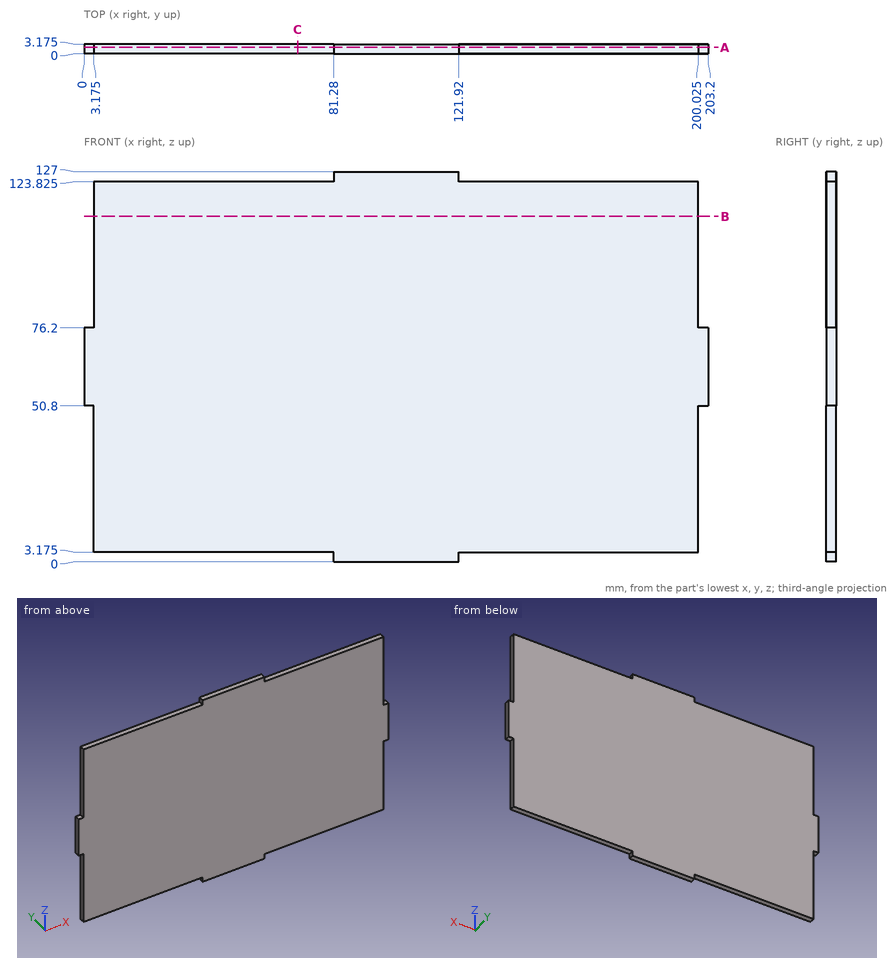
Part print with two shaded views. Sizes in mm from the minimum x, y, z corner. Coordinates: 2 decimals unless noted, no trailing zeros. Write each loop counter-clockwise with the first axis right and the second up, starting at its lowest first coordinate (ties: lowest second). Pieces come first, ordered by that corner, then holes.
(1) Pin check, flat tips, straight feed: pin 1 Ø8 at (x, z) = (45, 27.5) entering from -Y; pin 2 Ø1 at (x, y) = (31.5, 1.5) entering from -Z (3 decimals); pin 3 Ø1 at (x, y) = (2, 1) entering from +Z; pin 4 Ø1 at (y, z) = (1, 1.5) entering from +X. Stop position of each tip, or through.
(2) Cut at A-A on y = 2.1. List the corners of the cut face in (x, z) (3 decimals).
(3) Cut at C-C on x = 69.5. List the corners of the cut face in (y, z) (3 decimals), and give its area (3 significant figures).
(4) Cut at B-B on z = 112.5. List the corners of the cut face in (x, y) (3 decimals).
(5) Drill centre lines: line 1 (Z direction, x = 190, y = 1.75) (3 decimals); line 2 (X direction, y = 2.3, z = 46) (3 decimals). Where is each one in solid material? Low to high.
Working result:
1. pin 1: stops at y = 0
1. pin 2: stops at z = 3.175
1. pin 3: stops at z = 76.2
1. pin 4: stops at x = 121.92
2. outline: (0, 50.8) - (3.175, 50.8) - (3.175, 3.175) - (81.28, 3.175) - (81.28, 0) - (121.92, 0) - (121.92, 3.175) - (200.025, 3.175) - (200.025, 50.8) - (203.2, 50.8) - (203.2, 76.2) - (200.025, 76.2) - (200.025, 123.825) - (121.92, 123.825) - (121.92, 127) - (81.28, 127) - (81.28, 123.825) - (3.175, 123.825) - (3.175, 76.2) - (0, 76.2) - close
3. outline: (0, 3.175) - (3.175, 3.175) - (3.175, 123.825) - (0, 123.825) - close
3. area: 383 mm2
4. outline: (3.175, 0) - (200.025, 0) - (200.025, 3.175) - (3.175, 3.175) - close
5. line 1: z = 3.175 to 123.825
5. line 2: x = 3.175 to 200.025
